from build123d import *

# Parameters (mm, degrees)
SKETCH1_W           = 880
SKETCH1_H           = 36
BOSS_EXTRUDE1_DEPTH = 50
SKETCH2_W           = 30
SKETCH2_H           = 30
CUT_EXTRUDE1_DEPTH  = 50
SKETCH3_R           = 11
CUT_EXTRUDE2_DEPTH  = 50


with BuildPart() as part:
    # Sketch1 → Boss-Extrude1 (new body)
    with BuildSketch(Plane(origin=(0, 0, 0), x_dir=(1, 0, 0), z_dir=(0, 1, 0))):
        Rectangle(SKETCH1_W, SKETCH1_H)
    extrude(amount=BOSS_EXTRUDE1_DEPTH)

    # Sketch2 → Cut-Extrude1 (cut)
    with BuildSketch(Plane(origin=(0, 50, 0), x_dir=(1, 0, 0), z_dir=(0, 1, 0))):
        with Locations((-415, 0)):
            Rectangle(SKETCH2_W, SKETCH2_H)
        with Locations((415, 0)):
            Rectangle(SKETCH2_W, SKETCH2_H)
    extrude(amount=-CUT_EXTRUDE1_DEPTH, mode=Mode.SUBTRACT)

    # Sketch3 → Cut-Extrude2 (cut)
    with BuildSketch(Plane(origin=(0, 50, 0), x_dir=(1, 0, 0), z_dir=(0, 1, 0))):
        with Locations(Location((-40, 0, 0), (0, 0, 270))):
            Circle(SKETCH3_R)
        with Locations(Location((40, 0, 0), (0, 0, 270))):
            Circle(SKETCH3_R)
    extrude(amount=-CUT_EXTRUDE2_DEPTH, mode=Mode.SUBTRACT)


solid = part.part
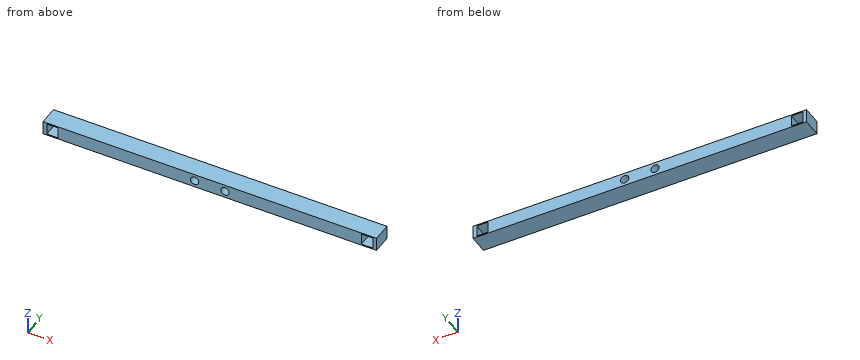
Part model, mm, in its own coordinate system. Give positions to 0.01 mm unless a question says otherwise; leave off trailing zeros. Loops run counter-clockwise (first coordinate to the right, second up) from the corner with the lowest first, then second, coordinate; pieces in that order, holes last. Notation, with made-up numbers: M 20.5,9.25 L 71.5,9.25 A18 cw 71.5,13.25 Z; hole C 27,-5 d4. An arc over 180 degrees is marked long. Put each result on its own line as item: value. Start each with the question number.
1) Saw through at A-A (z = 0). List the corners of the cut face in (x, y).
2) Flat gauge pin, fed straight in: pin 1 (4 mm diameter, centred on x = 70, z = 12.5, fed in from -Y). Where does the tip first touch, or does it go through?
3) Saw through at C-C (y = 28). List the corners of the cut face in (x, z).
4) Probe probe 1 along X at (y, z) = (24.5, -14); probe 2 along X at (y, z) = (12, 0); probe 3 along Z at (x, y) = (-403, 33.5). List the from-to ranges inside material, lowest first.
5) Saw through at B-B (x = 40). List the corners of the cut face in (y, z), then the cut area to 3 significant figures.
Numbers:
1. outline: M -440,0 L -430,0 L -430,50 L -440,50 Z; M -400,0 L -51,0 L -51,50 L -400,50 Z; M -29,0 L 29,0 L 29,50 L -29,50 Z; M 51,0 L 400,0 L 400,50 L 51,50 Z; M 430,0 L 440,0 L 440,50 L 430,50 Z
2. pin 1: y = 0
3. outline: M -440,-18 L 440,-18 L 440,18 L -440,18 Z; hole M -430,-15 L -400,-15 L -400,15 L -430,15 Z; hole C -40,0 d22; hole C 40,0 d22; hole M 400,-15 L 430,-15 L 430,15 L 400,15 Z
4. probe 1: -440 to -430, -400 to 400, 430 to 440
4. probe 2: -440 to -430, -400 to -51, -29 to 29, 51 to 400, 430 to 440
4. probe 3: -18 to -15, 15 to 18
5. outline: M 0,-18 L 50,-18 L 50,-11 L 0,-11 Z; M 0,11 L 50,11 L 50,18 L 0,18 Z
5. area: 700 mm^2
